```python
from build123d import *

# Parameters (mm, degrees)
BOSS_EXTRUDE1_DEPTH     = 0.35
SCALE1_SCALE            = 10
SKETCH2_R               = 4
CUT_EXTRUDE1_DEPTH      = 1
CUT_EXTRUDE1_DEPTH_BACK = 4.5


with BuildPart() as part:
    # Sketch1 → Boss-Extrude1 (new body)
    with BuildSketch(Plane(origin=(0, 0, 0), x_dir=(1, 0, 0), z_dir=(0, 1, 0))):
        with BuildLine():
            Line((-0.845785748, -19.220149774), (12.154214252, 2.13400673))
            Line((12.154214252, 2.13400673), (12.154214252, 26.456928478))
            ThreePointArc((12.154214252, 26.456928478), (1.891851134, 25.289168137), (-7.845785748, 21.84559602))
            Line((-7.845785748, 21.84559602), (-7.845785748, -19.220149774))
            Line((-7.845785748, -19.220149774), (-0.845785748, -19.220149774))
        make_face()
    extrude(amount=BOSS_EXTRUDE1_DEPTH)


with BuildPart() as part_1:
    # Scale1: scaled about (1.302109207, 0.175, -5.681101669)
    add(part.part.scale(SCALE1_SCALE).moved(Location((-11.718982863, -1.575, 51.129915021))))

    # Sketch2 → Cut-Extrude1 (cut, two sides)
    with BuildSketch(Plane(origin=(0, 1.925, 0), x_dir=(1, 0, 0), z_dir=(0, 1, 0))) as cut_extrude1_sk:
        with Locations((41.216468576, -33.118318866)):
            Circle(SKETCH2_R)
    extrude(amount=CUT_EXTRUDE1_DEPTH, mode=Mode.SUBTRACT)
    extrude(cut_extrude1_sk.sketch, amount=-CUT_EXTRUDE1_DEPTH_BACK, mode=Mode.SUBTRACT)


solid = part_1.part
```
Verification items for the finished model (mm, model axes). Round coordinates to 2 decimals unless told otherwise and drop trailing zeros. Order: outer loops, then holes, each group sorted by start corner. A loop starts at its lowest first (then second) coordinate and runs counter-clockwise, first axis right, second up. Notation, with made-up numbers: (-19, -10) - (0, -10) arc R13 cw to (0, 5) - close; hole circle Ø9 at (-35, -27). An arc over 180 degrees is marked (long way). Use CSV: the item, a comma, the result in double quotes. Start each with the question number.
1) Go/stop test with a flat-tipped pin: P1, Ø1, axis at x = 4, y = 1, coming from the +Z side. Record where the tip stops, or that it passes through.
2) Mould release check, pull along X, two halves, no side actions. Record for faces 1 (the flat face through (43.91, 0.15, 138.06)), 2 (the cylindrical face through (8.612, 0.151, -202.085)), 3 (the flat face through (8, -1.575, 12)), 4 (the cylindrical face through (38.04, 0.2, 35.55)): +X half, -X half, draft (parallel to the pull), parting line (faces both ways), or undercut.
3) Section check B-B, the plane z = 108. Record the cut outline in (x, y) (3 decimals), plus the area to 3 significant figures.
4) Section check A-A, the plane y = 0.3. Record the cut outline in (x, z).
5) Thickness scan on L1, parallel to X at y = 1.1, z = 143.5; L2, parallel to Z at x = 4, y = -0.55; L3, parallel to Z at x = -8.5, y = 1. Record the ranges inside material, lowest first.
6) Section check C-C, the plane x = 5. Record the cut outline in (y, z) (3 decimals).
Answers:
1,P1,"stops at z = 204.44"
2,face 1,"+X half"
2,face 2,"-X half"
2,face 3,"draft"
2,face 4,"undercut"
3,outline,"(-90.177, -1.575) - (62.21, -1.575) - (62.21, 1.925) - (-90.177, 1.925) - close"
3,area,"533 mm²"
4,outline,"(-90.18, -167.33) arc R456.77 ccw to (109.82, -213.44) - (109.82, 29.79) - (-20.18, 243.33) - (-90.18, 243.33) - close; hole circle Ø8 at (41.22, 33.12)"
5,L1,"x = -90.18 to 40.6"
5,L2,"z = -201.01 to 203.62"
5,L3,"z = -197.85 to 224.15"
6,outline,"(-1.575, -201.249) - (1.925, -201.249) - (1.925, 201.975) - (-1.575, 201.975) - close"
